```python
from build123d import *

# Parameters (mm, degrees)
SKETCH2_R           = 10.025
BOSS_EXTRUDE1_DEPTH = 2
SKETCH3_W           = 2
SKETCH3_H           = 15.533622691
CUT_EXTRUDE1_DEPTH  = 8.525


with BuildPart() as part:
    # Sketch1 → Revolve1 (revolve)
    with BuildSketch(Plane.XY):
        with BuildLine():
            Line((9.525, 0), (0, 0))
            Line((0, 0), (0, 9.525))
            ThreePointArc((0, 9.525), (6.735192091, 6.735192091), (9.525, 0))
        make_face()
    revolve(axis=Axis((0, 0, 0), (0, 1, 0)))

    # Sketch2 → Boss-Extrude1 (add)
    with BuildSketch(Plane.XZ):
        Circle(SKETCH2_R)
    extrude(amount=-BOSS_EXTRUDE1_DEPTH)

    # Sketch3 → Cut-Extrude1 (cut, through all)
    with BuildSketch(Plane(origin=(0, 2, 0), x_dir=(1, 0, 0), z_dir=(0, 1, 0))):
        Polygon((-9.533657483, -3.1), (9.533657483, -3.1), (10.025, -3.1), (10.025, 3.1), (9.533657483, 3.1), (-9.533657483, 3.1), (-10.025, 3.1), (-10.025, -3.1), align=None)
        with Locations((0, -12.866811346)):
            Rectangle(SKETCH3_W, SKETCH3_H)
        with Locations((0, 12.866811346)):
            Rectangle(SKETCH3_W, SKETCH3_H)
        with Locations((4, -12.866811346)):
            Rectangle(SKETCH3_W, SKETCH3_H)
        with Locations((4, 12.866811346)):
            Rectangle(SKETCH3_W, SKETCH3_H)
        with Locations((8, -12.866811346)):
            Rectangle(SKETCH3_W, SKETCH3_H)
        with Locations((8, 12.866811346)):
            Rectangle(SKETCH3_W, SKETCH3_H)
        with Locations((12, -12.866811346)):
            Rectangle(SKETCH3_W, SKETCH3_H)
        with Locations((12, 12.866811346)):
            Rectangle(SKETCH3_W, SKETCH3_H)
        with Locations((16, -12.866811346)):
            Rectangle(SKETCH3_W, SKETCH3_H)
        with Locations((16, 12.866811346)):
            Rectangle(SKETCH3_W, SKETCH3_H)
        with Locations((-4, 12.866811346)):
            Rectangle(SKETCH3_W, SKETCH3_H)
        with Locations((-4, -12.866811346)):
            Rectangle(SKETCH3_W, SKETCH3_H)
        with Locations((-8, 12.866811346)):
            Rectangle(SKETCH3_W, SKETCH3_H)
        with Locations((-8, -12.866811346)):
            Rectangle(SKETCH3_W, SKETCH3_H)
        with Locations((-12, 12.866811346)):
            Rectangle(SKETCH3_W, SKETCH3_H)
        with Locations((-12, -12.866811346)):
            Rectangle(SKETCH3_W, SKETCH3_H)
        with Locations((-16, 12.866811346)):
            Rectangle(SKETCH3_W, SKETCH3_H)
        with Locations((-16, -12.866811346)):
            Rectangle(SKETCH3_W, SKETCH3_H)
    extrude(amount=CUT_EXTRUDE1_DEPTH, mode=Mode.SUBTRACT)


solid = part.part
```
The model under review builds one solid part; all positions refer to its coordinate system, in mm. A direction names the side the tool comes from. Give positions to 0.01 mm unless a question says otherwise; leave off trailing zeros. Write each loop counter-clockwise with the first axis right and the second up, starting at its lowest first coordinate (ties: lowest second). Pieces come first, ordered by that corner, then holes. Notation, with made-up numbers: (24.25, 54) -> (37.25, 54) arc R14 ccw to (37.25, 72) -> close; hole circle Ø9 at (23.5, 21). An arc over 180 degrees is marked (long way). Answer in a Markdown table with one row per item.
1) Add section A-A on x = 0. State the section outline as (y, z) points (3 decimals).
Worked answers:
| item | result |
|---|---|
| outline | (0, -10.025) -> (2, -10.025) -> (2, -5.1) -> (8.045, -5.1) arc R9.525 ccw to (9.006, -3.1) -> (2, -3.1) -> (2, 3.1) -> (9.006, 3.1) arc R9.525 ccw to (8.045, 5.1) -> (2, 5.1) -> (2, 10.025) -> (0, 10.025) -> close |
2) Add section C-C on y = 1.5. State the section outline as (x, z) points (3 decimals), plus the area to 3 significant figures.
Worked answers:
| item | result |
|---|---|
| outline | circle Ø20.05 at (0, 0) |
| area | 316 mm² |
3) Add section D-D on z = 0. State the section outline as (x, y) points (3 decimals).
Worked answers:
| item | result |
|---|---|
| outline | (-10.025, 0) -> (10.025, 0) -> (10.025, 2) -> (-10.025, 2) -> close |
4) Tool access review of faces 1 (the flat face through (4, 5, 5.1)), 2 (the flat face through (7, 2.8, -5.5)), 3 (the flat face through (-7, 2.8, -5.5)), 4 (the flat face through (4, 5, -5.1)), 5 (the flat face through (0, 2, 0)): name each direction out of +Z, -Z, +X, -X, +Y, -Y from which nothing blocks a thin tool from reaching the whole face with its end or side.
Worked answers:
| item | result |
|---|---|
| face 1 | +Z, +Y |
| face 2 | -Z, +X, +Y |
| face 3 | -Z, -X, +Y |
| face 4 | -Z, +Y |
| face 5 | +Y |
5) For L1, parallel to X at y = 2.75, z = -5.25; L2, parallel to Z at x = 0, y = 3.75; L3, parallel to X at y = 2.25, z = 6.25, list the stretches that pass through material, from the lowest coordinate up. Write a range as [from, to].
Worked answers:
| item | result |
|---|---|
| L1 | [-7, -5], [-3, -1], [1, 3], [5, 7] |
| L2 | [-5.1, -3.1], [3.1, 5.1] |
| L3 | [-6.83, -5], [-3, -1], [1, 3], [5, 6.83] |
6) Mouldability with a two-part tool opening along Z and no side actions: class faces 6 (the flat face through (0, 5, 3.1)), 7 (the flat face through (-5, 4, -6)), 8 (the flat face through (0, 5, -3.1)), 9 (the flat face through (-4, 5, -5.1)) as +Z half, -Z half, draft (parallel to the pull), parting line (faces both ways), or undercut.
Worked answers:
| item | result |
|---|---|
| face 6 | undercut |
| face 7 | draft |
| face 8 | undercut |
| face 9 | -Z half |
7) Clearance check with flat-ended pins moving along their axes: P1, Ø2, axis at y = 4, z = 8, coming from the +X side; P2, Ø1, axis at y = 6, z = 1, coming from the -X side; P3, Ø5, axis at x = -4, y = 5.5, coming from the -Z side; P4, Ø4, axis at y = 3.5, z = -6, coming from the -X side. State where each tip first meets the part, or that it passes through.
Worked answers:
| item | result |
|---|---|
| P1 | x = 5.25 |
| P2 | through |
| P3 | z = -8.5 |
| P4 | x = -8.87 |
8) Add section B-B on y = 7. State the section outline as (x, z) points, plus the area to 3 significant figures.
Worked answers:
| item | result |
|---|---|
| outline | (-5.67, -3.1) arc R6.46 ccw to (-3.96, -5.1) -> (-3, -5.1) -> (-3, -5.72) arc R6.46 ccw to (-1, -6.38) -> (-1, -5.1) -> (1, -5.1) -> (1, -6.38) arc R6.46 ccw to (3, -5.72) -> (3, -5.1) -> (3.96, -5.1) arc R6.46 ccw to (5.67, -3.1) -> close; (-5.67, 3.1) -> (5.67, 3.1) arc R6.46 ccw to (3.96, 5.1) -> (3, 5.1) -> (3, 5.72) arc R6.46 ccw to (1, 6.38) -> (1, 5.1) -> (-1, 5.1) -> (-1, 6.38) arc R6.46 ccw to (-3, 5.72) -> (-3, 5.1) -> (-3.96, 5.1) arc R6.46 ccw to start |
| area | 47.6 mm² |
